```python
from build123d import *

# Parameters (mm, degrees)
F0_W     = 70
F0_H     = 20
F0_R     = 2.5
F1_DEPTH = 3
F2_R     = 5
F3_DEPTH = 110


with BuildPart() as f1:
    # F0 (on Front) → F1 (new body)
    with BuildSketch(Plane.XZ):
        Rectangle(F0_W, F0_H)
        with Locations((-25, 0)):
            Circle(F0_R, mode=Mode.SUBTRACT)
        with Locations((25, 0)):
            Circle(F0_R, mode=Mode.SUBTRACT)
    extrude(amount=F1_DEPTH)

    # F2 (on face) → F3 (join)
    with BuildSketch(Plane.XZ.offset(3)):
        Circle(F2_R)
    extrude(amount=F3_DEPTH)


solid = f1.part
```
Geometry check sheet. Reference: the model listing, model coordinates, mm. A direction names the side the tool comes from. Give positions to 0.01 mm unless a question says otherwise; leave off trailing zeros. Write each loop counter-clockwise with the first axis right and the second up, starting at its lowest first coordinate (ties: lowest second). Pieces come first, ordered by that corner, then holes.
1) Access from +Z, -Z, +X, -X, +Y, -Y to the whole of each face (thin tool, end or side, straight path). Record for faces 4 (the flat face through (0, -113, 0)), 5 (the cylindrical face through (-1.08, -57.23, -4.88)).
2) Section check A-A, the plane x = 25. Record the boundary of the cut face in (y, z).
3) Gauge pin test, flat ends, axial feed: pin 1 (6 mm diameter, centred on y = -88.5, z = 1.5, fed in from +X); pin 2 (1 mm diameter, centred on x = -15, z = 7.5, fed in from -Y); pin 3 (4 mm diameter, centred on x = -0.5, y = -66.5, fed in from +Z). Record the tip position at first contact, or that the pin passes through.
4) Section check D-D, the plane y = -52.5. Record the boundary of the cut face in (x, z), and give its area (3 significant figures).
5) Release check for a two-part mould opening along Z. For faces 1 (the flat face through (35, -1, 0)), 2 (the cylindrical face through (22.5, -1.5, 0.1)), 3 (the flat face through (0, -1, -10)) record: pulls with the +Z half, pulls with the -Z half, needs draft (parallel to the pull), parting line crosses it, or undercut.
6) Section check B-B, the plane z = 0. Record the boundary of the cut face in (x, y), and give its area (3 significant figures).
7) Section check C-C, the plane x = 0. Record the boundary of the cut face in (y, z), and give its area (3 significant figures).
8) Material ranges on L1, parallel to Y at x = -27, z = 6.5; L2, parallel to X at y = -26, z = 0.5; L3, parallel to X at y = -60.5, z = 1, recorded low to high.
Computed:
1. face 4: +Z, -Z, +X, -X, -Y
1. face 5: -Y
2. outline: (-3, -10) - (0, -10) - (0, -2.5) - (-3, -2.5) - close; (-3, 2.5) - (0, 2.5) - (0, 10) - (-3, 10) - close
3. pin 1: stops at x = 5
3. pin 2: stops at y = -3
3. pin 3: stops at z = 5
4. outline: circle Ø10 at (0, 0)
4. area: 78.5 mm2
5. face 1: needs draft
5. face 2: undercut
5. face 3: pulls with the -Z half
6. outline: (-35, -3) - (-27.5, -3) - (-27.5, 0) - (-35, 0) - close; (-22.5, -3) - (-5, -3) - (-5, -113) - (5, -113) - (5, -3) - (22.5, -3) - (22.5, 0) - (-22.5, 0) - close; (27.5, -3) - (35, -3) - (35, 0) - (27.5, 0) - close
6. area: 1,280 mm2
7. outline: (-113, -5) - (-3, -5) - (-3, -10) - (0, -10) - (0, 10) - (-3, 10) - (-3, 5) - (-113, 5) - close
7. area: 1,160 mm2
8. L1: y = -3 to 0
8. L2: x = -4.97 to 4.97
8. L3: x = -4.9 to 4.9
